The model under review builds one solid part; all positions refer to its coordinate system, in mm. Face numbers are marked on the shaded views. A direction names the side the tool comes from. Coordinates: 2 decimals unless noted, no trailing zeros. Order: outer loops, then holes, each group sorted by start corner. A loop starts at its lowest first (then second) coordinate and runs counter-clockwise, first axis right, second up. Notation, with made-up numbers: M -31.75,-27.75 L 8.25,-27.75 A22 ccw 8.25,-11.75 Z; hole C 31.25,1.25 d2. An arc over 180 degrees is marked long. Answer in a Markdown table with one row per item.
Autodesk Inventor part; units mm, degrees
ref_plane "YZ Plane" through (0, 0, 0) normal (1, 0, 0) x (0, 1, 0)
ref_plane "XZ Plane" through (0, 0, 0) normal (0, 1, 0) x (-1, 0, 0)
ref_plane "XY Plane" through (0, 0, 0) normal (0, 0, 1) x (1, 0, 0)
sketch "Sketch1" plane through (0, 0, 0) normal (0, 1, 0) x (-1, 0, 0)
  line L0 (0, 0) -> (-20.32, 0)
  line L1 (-20.32, 0) -> (-20.32, -76.2)
  line L2 (-20.32, -76.2) -> (0, -76.2)
  line L3 (0, -76.2) -> (0, 0)
  dimension "d0" = 20.32
  dimension "d1" = 76.2
extrude "Extrusion1" add sketch "Sketch1" along normal blind 7.62
sketch "Sketch2" plane through (0, 7.62, 0) normal (0, 1, 0) x (1, 0, 0)
  line L0 (0, 0) -> (0, 12.7)
  line L1 (0, 76.2) -> (0, 0)
  line L2 (20.32, 0) -> (20.32, 76.2)
  line L3 (0, 12.7) -> (20.32, 12.7)
  line L4 (20.32, 12.7) -> (20.32, 63.5)
  line L5 (20.32, 63.5) -> (0, 63.5)
  line L6 (0, 63.5) -> (0, 12.7)
  dimension "d4" = 12.7
  dimension "d5" = 50.8
extrude "Extrusion2" add sketch "Sketch2" along normal blind 50.8
sketch "Sketch3" plane through (20.32, 0, 0) normal (1, 0, 0) x (0, 0, -1)
  line L0 (12.7, 58.42) -> (63.5, 58.42)
  line L1 (38.1, 58.42) -> (38.1, 33.02)
  circle A0 centre (38.1, 33.02) radius 19.05
  point P0 (0, 0)
  dimension "d8" = 25.4
  dimension "d9" = 38.1
extrude "Extrusion3" cut sketch "Sketch3" against normal blind 15.24
sketch "Sketch4" plane through (5.08, 33.02, -38.1) normal (1, 0, 0) x (0, 0, -1)
  circle A0 centre (0, 0) radius 19.05
  line L0 (0, 19.05) -> (0, 12.7)
  line L1 (0, 12.7) -> (0, 6.35)
  circle A1 centre (0, 6.35) radius 6.35
  point P0 (-38.1, -33.02)
  dimension "d12" = 6.35
  dimension "d13" = 6.35
  dimension "d14" = 12.7
extrude "Extrusion4" cut sketch "Sketch4" against normal blind 5.08 contours A1
sketch "Sketch5" plane through (5.08, 33.02, -38.1) normal (1, 0, 0) x (0, 0, -1)
  circle A0 centre (0, 6.35) radius 6.35
  point P0 (-38.1, -33.02)
  point P1 (0, 0)
pattern_circular "Circular Pattern1" count 6 over 360 about axis through (5.08, 33.02, -38.1) along (1, 0, 0) of "Extrusion4"
fillet "Fillet1" radius 25.4 1 edges at (10.16, 58.42, -12.7)
fillet "Fillet2" radius 25.4 1 edges at (10.16, 58.42, -63.5)
sketch "Sketch6" plane through (0, 7.62, 0) normal (0, 1, 0) x (1, 0, 0)
  line L0 (0, 12.7) -> (20.32, 12.7)
  line L1 (10.16, 12.7) -> (10.16, 2.54)
  line L2 (10.16, 12.7) -> (10.16, 7.62)
  line L3 (0, 63.5) -> (20.32, 63.5)
  line L4 (10.16, 63.5) -> (10.16, 68.58)
  circle A0 centre (10.16, 7.62) radius 2.54
  circle A1 centre (10.16, 68.58) radius 2.54
  point P0 (0, 0)
  dimension "d24" = 10.16
  dimension "d25" = 5.08
  dimension "d26" = 5.08
  dimension "d27" = 5.08
  dimension "d28" = 5.08
fillet "Fillet5" radius 25.4 2 edges at (10.16, 7.62, -63.5) (10.16, 7.62, -12.7)
hole "Hole1" at (10.16, 7.62, -7.62) at (10.16, 7.62, -68.58) direction (0, -1, 0) diameter 5.08 end through all counterbore diameter 10.16 counterbore depth 3.81
sketch "Sketch8" plane through (10.16, 7.62, -7.62) normal (0, -1, 0) x (1, 0, 0)
  circle A0 centre (0, 0) radius 5.08
  circle A1 centre (0, -60.96) radius 2.54
  line L0 (-2.54, -60.96) -> (0, -60.96)
  circle A2 centre (0, -60.96) radius 5.08
  point P0 (-10.16, 7.62)
  dimension "d37" = 10.16
  dimension "d38" = 10.16
extrude "Extrusion5" cut sketch "Sketch8" against normal blind 25.4 contours A0 | A1 | A2
sketch "Sketch9" plane through (5.08, 33.02, -38.1) normal (1, 0, 0) x (0, 0, -1)
  arc A0 (5.4993, 9.525) -> (-5.4993, 9.525) centre (0, 6.35) ccw
  arc A1 (-5.4993, -9.525) -> (5.4993, -9.525) centre (0, -6.35) ccw
  point P0 (-38.1, -33.02)
  point P1 (0, 12.7)
  point P2 (0, -12.7)
properties part number "Motor Mount V1"
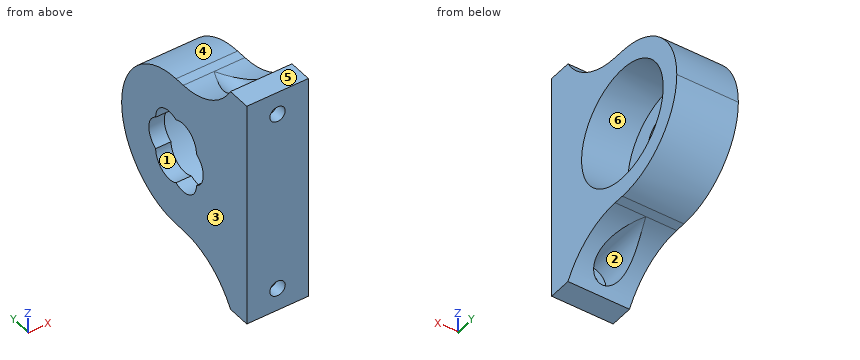
(1) Take a section at D-D (y = 37.5). Write out the cut boundary in (x, z).
Report:
| item | result |
|---|---|
| outline | M 0,-63.1 L 20.32,-63.1 L 20.32,-56.62 L 5.08,-56.62 L 5.08,-49.81 L 0,-49.81 Z; M 0,-26.39 L 5.08,-26.39 L 5.08,-19.58 L 20.32,-19.58 L 20.32,-13.1 L 0,-13.1 Z |
(2) Insertion check: P1, Ø6, axis at x = 5, y = 49, coming from the +Z side; P2, Ø8, axis at x = 10.16, z = -7.62, coming from the +Y side; P3, Ø2, axis at x = 7.5, y = 22.5, coming from the -Z side; P4, Ø4.5, axis at x = 10.16, z = -68.58, coming from the +Y side. Each pin has a flat end and moves straight along its axis. Give the tip position at first contact, or say it passes through.
Report:
| item | result |
|---|---|
| P1 | z = -16.27 |
| P2 | y = 3.81 |
| P3 | z = -64.75 |
| P4 | through |
(3) Take a section at C-C (y = 9). Write out the cut boundary in (x, z).
Report:
| item | result |
|---|---|
| outline | M 0,-74.06 L 20.32,-74.06 L 20.32,-2.14 L 0,-2.14 Z; hole C 10.16,-68.58 d10.16; hole C 10.16,-7.62 d10.16 |
(4) Take a section at A-A (x = 11.25). State how many separate pieces and enclosed holes the cut face has, then the cut area to 3 significant figures.
Report:
| item | result |
|---|---|
| separate pieces | 3 |
| enclosed holes | 1 |
| area | 1,640 mm^2 |
(5) Machinability: for the marked faces 1, 2 and 3, which of the approach directions +Z, -Z, +X, -X, +Y, -Y give a long, thin tool a straight path to every point of the face, cutting with its end or side? Answer none if there is none.
Report:
| item | result |
|---|---|
| face 1 | +X, -X |
| face 2 | +Y |
| face 3 | +Z, -Z, -X, +Y, -Y |
(6) Take a section at B-B (z = -7.62). Write out the cut boundary in (x, y), then the cut area to 3 significant figures.
Report:
| item | result |
|---|---|
| outline | M 0,0 L 7.62,0 L 7.62,3.81 L 5.08,3.81 L 5.08,14.38 L 0,14.38 Z; M 12.7,0 L 20.32,0 L 20.32,14.38 L 15.24,14.38 L 15.24,3.81 L 12.7,3.81 Z |
| area | 165 mm^2 |
(7) The part is to be moulded in two halves that separate along Y. For the marked faces 4, 5 and 6, say which applies: +Y half, -Y half, draft (parallel to the pull), parting line (faces both ways), or undercut.
Report:
| item | result |
|---|---|
| face 4 | +Y half |
| face 5 | draft |
| face 6 | undercut |
(8) To check wall thickness, follow line 1 (Z direction, x = 10.16, y = 2.1); line 2 (X direction, y = 2.25, z = -68.58); line 3 (Z direction, x = 17.5, y = 33.5). State the ranges of each line that lie inside material, in increasing order. Write a range as [from, to].
Report:
| item | result |
|---|---|
| line 1 | [-76.2, -71.12], [-66.04, -10.16], [-5.08, 0] |
| line 2 | [0, 7.62], [12.7, 20.32] |
| line 3 | [-63.5, -57.14], [-19.06, -12.7] |
